The listing builds one solid part. Answer for the finished solid, in the listing's coordinates (mm). A direction names the side the tool comes from. Give positions to 0.01 mm unless a question says otherwise; leave off trailing zeros. Answer as CSV lines item,"result". Start each with the question number.
1. Flat-ended cylindrical pins translate along their axes: pin 1 (0.7 mm diameter, centred on x = -54, y = -72, fed in from +Z); pin 2 (3 mm diameter, centred on x = -64, y = -115, fed in from -Z); pin 3 (5 mm diameter, centred on y = -142, z = 30.5, fed in from -X); pin 4 (5 mm diameter, centred on y = -181.5, z = 15, fed in from -X). Find the tip coordinate at first contact, or state that the pin passes through.
2. Determine the mould class of faces 4 (the flat face through (-88.87, -125.22, 14.16)), 5 (the flat face through (-59.773, -125.222, 5.735)), 6 (the flat face through (-59.62, -125.222, 43.262)) for opening direction Z: +Z half, -Z half, draft (parallel to the pull), parting line (faces both ways), or undercut.
3. Which of the six approach directions +Z, -Z, +X, -X, +Y, -Y give full straight-line access (tool end or side, diameter ignored) to faces 1 (the cylindrical face through (-66.3, -125.2, 32.4)), 2 (the flat face through (-80.447, -125.222, 43.254)), 3 (the flat face through (-88.878, -125.222, 34.984))?
4. Consider line 1 along X through (y, z) = (-206, 9); line 2 along Z through (x, y) = (-80.5, -129.5); line 3 along X through (y, z) = (-162, 18.5). Determine where each line is inside the solid, lowest interval first. Write a range as [from, to].
from build123d import *

# Parameters (mm, degrees)
F1_DEPTH = 254


# Not quite as in the source:
# - ends of sketch curves that miss each other by under 0.0002 mm in the source are joined


with BuildPart() as f1:
    # F0 (on Front) → F1 (new body)
    with BuildSketch(Plane.XZ):
        with BuildLine():
            Line((-51.0604008, 40.36949), (-54.2354008, 43.5444646))
            Line((-54.2354008, 43.5444646), (-65.158493, 42.9719994))
            Line((-65.158493, 42.9719994), (-65.9448008, 42.1434006))
            Line((-65.9448008, 42.1434006), (-65.9448008, 39.9630646))
            Line((-65.9448008, 39.9630646), (-65.1573754, 39.17569))
            Line((-65.1573754, 39.17569), (-60.3517716, 39.17569))
            ThreePointArc((-60.3517716, 39.17569), (-59.6477719597, 38.7052864789), (-59.8129689327, 37.8748619331))
            Line((-59.8129689327, 37.8748619331), (-63.1878848, 34.4999818))
            ThreePointArc((-63.1878848, 34.4999818), (-66.3629880966, 32.3740308419), (-70.1104008, 31.6271402404))
            ThreePointArc((-70.1104008, 31.6271402404), (-73.8578286035, 32.3740244671), (-77.0329470659, 34.4999769462))
            Line((-77.0329470659, 34.4999769462), (-80.4078656, 37.8748544))
            ThreePointArc((-80.4078656, 37.8748544), (-80.5730550403, 38.7052864789), (-79.8690554, 39.17569))
            Line((-79.8690554, 39.17569), (-75.0634516, 39.17569))
            Line((-75.0634516, 39.17569), (-74.2760262, 39.9630646))
            Line((-74.2760262, 39.9630646), (-74.2760262, 42.1434006))
            Line((-74.2760262, 42.1434006), (-75.062334, 42.9719994))
            Line((-75.062334, 42.9719994), (-85.9854008, 43.5444646))
            Line((-85.9854008, 43.5444646), (-89.1604008, 40.36949))
            Line((-89.1604008, 40.36949), (-88.5879356, 29.4463978))
            Line((-88.5879356, 29.4463978), (-87.7593368, 28.66009))
            Line((-87.7593368, 28.66009), (-85.5790008, 28.66009))
            Line((-85.5790008, 28.66009), (-84.7916262, 29.4475154))
            Line((-84.7916262, 29.4475154), (-84.7916262, 34.2531192))
            ThreePointArc((-84.7916262, 34.2531192), (-84.3212226789, 34.9571188403), (-83.4907981331, 34.7919218673))
            Line((-83.4907981331, 34.7919218673), (-80.115918, 31.417006))
            ThreePointArc((-80.115918, 31.417006), (-77.9899670419, 28.2419027034), (-77.2430764404, 24.49449))
            ThreePointArc((-77.2430764404, 24.49449), (-77.9899606671, 20.7470621965), (-80.1159131462, 17.5719437341))
            Line((-80.1159131462, 17.5719437341), (-83.4907906, 14.1970252))
            ThreePointArc((-83.4907906, 14.1970252), (-84.3212226789, 14.0318357597), (-84.7916262, 14.7358354))
            Line((-84.7916262, 14.7358354), (-84.7916262, 19.5414392))
            Line((-84.7916262, 19.5414392), (-85.5790008, 20.3288646))
            Line((-85.5790008, 20.3288646), (-87.7593368, 20.3288646))
            Line((-87.7593368, 20.3288646), (-88.5879864, 19.5425314))
            Line((-88.5879864, 19.5425314), (-89.1604262, 8.61949))
            Line((-89.1604262, 8.61949), (-85.9854262, 5.44449))
            Line((-85.9854262, 5.44449), (-75.062334, 6.0169552))
            Line((-75.062334, 6.0169552), (-74.2760262, 6.845554))
            Line((-74.2760262, 6.845554), (-74.2760262, 9.02589))
            Line((-74.2760262, 9.02589), (-75.0634516, 9.8132646))
            Line((-75.0634516, 9.8132646), (-79.8690554, 9.8132646))
            ThreePointArc((-79.8690554, 9.8132646), (-80.5730550403, 10.2836681211), (-80.4078580673, 11.1140926669))
            Line((-80.4078580673, 11.1140926669), (-77.0329422, 14.4889728))
            ThreePointArc((-77.0329422, 14.4889728), (-73.8578286035, 16.6149301329), (-70.1104008, 17.3618143619))
            ThreePointArc((-70.1104008, 17.3618143619), (-66.3629880966, 16.6149237581), (-63.187885217, 14.488972384))
            Line((-63.187885217, 14.488972384), (-59.8129614, 11.1141002))
            ThreePointArc((-59.8129614, 11.1141002), (-59.6477719597, 10.2836681211), (-60.3517716, 9.8132646))
            Line((-60.3517716, 9.8132646), (-65.1573754, 9.8132646))
            Line((-65.1573754, 9.8132646), (-65.9448008, 9.02589))
            Line((-65.9448008, 9.02589), (-65.9448008, 6.845554))
            Line((-65.9448008, 6.845554), (-65.158493, 6.0169552))
            Line((-65.158493, 6.0169552), (-54.2354008, 5.44449))
            Line((-54.2354008, 5.44449), (-51.0604008, 8.61949))
            Line((-51.0604008, 8.61949), (-51.6328406, 19.5425314))
            Line((-51.6328406, 19.5425314), (-52.4614902, 20.3288646))
            Line((-52.4614902, 20.3288646), (-54.6418262, 20.3288646))
            Line((-54.6418262, 20.3288646), (-55.4292008, 19.5414392))
            Line((-55.4292008, 19.5414392), (-55.4292008, 14.7358354))
            ThreePointArc((-55.4292008, 14.7358354), (-55.8996043211, 14.0318357597), (-56.7300288669, 14.1970327327))
            Line((-56.7300288669, 14.1970327327), (-60.104909, 17.5719486))
            ThreePointArc((-60.104909, 17.5719486), (-62.2308663329, 20.7470621965), (-62.9777505619, 24.49449))
            ThreePointArc((-62.9777505619, 24.49449), (-62.2308599581, 28.2419027034), (-60.104908584, 31.417005583))
            Line((-60.104908584, 31.417005583), (-56.7300364, 34.7919294))
            ThreePointArc((-56.7300364, 34.7919294), (-55.8996043211, 34.9571188403), (-55.4292008, 34.2531192))
            Line((-55.4292008, 34.2531192), (-55.4292008, 29.4475154))
            Line((-55.4292008, 29.4475154), (-54.6418262, 28.66009))
            Line((-54.6418262, 28.66009), (-52.4614902, 28.66009))
            Line((-52.4614902, 28.66009), (-51.6328406, 29.4464232))
            Line((-51.6328406, 29.4464232), (-51.0604008, 40.36949))
        make_face()
        with BuildLine():
            ThreePointArc((-73.497059, 24.49449), (-70.1104008, 27.8811482), (-66.7237426, 24.49449))
            ThreePointArc((-66.7237426, 24.49449), (-70.1104008, 21.1078318), (-73.497059, 24.49449))
        make_face(mode=Mode.SUBTRACT)
    extrude(amount=F1_DEPTH)


solid = f1.part
Checks:
1,pin 1,"stops at z = 43.54"
1,pin 2,"stops at z = 5.88"
1,pin 3,"stops at x = -88.77"
1,pin 4,"stops at x = -88.96"
2,face 4,"undercut"
2,face 5,"-Z half"
2,face 6,"+Z half"
3,face 1,"+Y, -Y"
3,face 2,"+Z, +Y, -Y"
3,face 3,"-X, +Y, -Y"
4,line 1,"x = [-89.14, -74.28], [-65.94, -51.08]"
4,line 2,"z = [5.73, 10.15], [11, 17.19], [31.8, 37.99], [38.84, 43.26]"
4,line 3,"x = [-88.64, -84.79], [-79.3, -60.92], [-55.43, -51.58]"
